Build history of the part. All positions in model axes, mm. Face numbers are marked on the shaded views. A direction names the side the tool comes from. Give positions to 0.01 mm unless a question says otherwise; leave off trailing zeros. Order: outer loops, then holes, each group sorted by start corner. A loop starts at its lowest first (then second) coordinate and runs counter-clockwise, first axis right, second up. Notation, with made-up numbers: (43, -29) -> (47, -29) arc R28 cw to (47, -5) -> close; hole circle Ø11 at (53, -22.75). An arc over 180 degrees is marked (long way). One line per question, with ' | ' between items. Start each with the question number.
(1) Cut at C-C (x = 62.5). Give the cut face in (y, z), then the cut area to 3 significant figures.
(2) Drill centre lines: L1, parallel to Y at x = -62, z = 8.5; L2, parallel to Z at x = -59, y = 38; L3, parallel to Z at x = 47.5, y = -47. Where is each one in solid material? Low to high. Write a range as from..to.
(3) Pin check, flat tips, straight feed: pin 1 Ø20 at (x, y) = (9, -26.5) entering from -Z; pin 2 Ø4.5 at (x, z) = (-2, 1.5) entering from -Y; pin 3 Ø16 at (x, y) = (93.5, 235) entering from +Z; pin 4 Ø6 at (y, z) = (109, -4) entering from +X. Stop position of each tip, or through.
(4) Cut at B-B (y = 129.5). Give the cut face in (x, z).
(5) Cut at A-A (z = -61). Give the cut face in (x, y).
(6) Cut at D-D (y = -14). Give the cut face in (x, z).
(7) Which spindle directions (+Z, -Z, +X, -X, +Y, -Y) get a long thin tool onto all of the face, cutting with end or side? Do the marked faces 1, 2, 3 and 4. Say none if no direction does.
from build123d import *

# Parameters (mm, degrees)
EXTRUDE_1_DEPTH = 4
SKETCH_11_W     = 156
SKETCH_11_H     = 90
EXTRUDE_2_DEPTH = 20
SKETCH_12_W     = 38
SKETCH_12_H     = 4
SKETCH_14_W     = 38
SKETCH_14_H     = 50
EXTRUDE_3_DEPTH = 20


with BuildPart() as part:
    # 草图1 → 凸台-拉伸1 (new body)
    with BuildSketch(Plane.XY):
        Polygon((-40, 0), (40, 0), (40, -160), (78, -160), (78, 0), (78, 50), (118, 90), (80, 90), (40, 50), (-40, 50), (-80, 90), (-118, 90), (-78, 50), (-78, 0), (-78, -160), (-40, -160), align=None)
    extrude(amount=EXTRUDE_1_DEPTH)

    # 草图11 → 凸台-拉伸2 (add)
    with BuildSketch(Plane.XY.offset(4)):
        with Locations((0, 5)):
            Rectangle(SKETCH_11_W, SKETCH_11_H)
    extrude(amount=EXTRUDE_2_DEPTH)

    # 扫描1: sweep along a path in 草图13
    with BuildLine(Plane(origin=(78, 0, 0), x_dir=(0, 0, -1), z_dir=(1, 0, 0))) as sweep_1_path:
        Line((-4, 90), (-4, 150))
        Line((-4, 150), (41, 227.942286341))
        Line((41, 227.942286341), (131, 227.942286341))
    # 草图12 → 扫描1 (sweep)
    with BuildSketch(Plane(origin=(0, 90, 0), x_dir=(1, 0, 0), z_dir=(0, 1, 0))):
        with Locations((-99, -2)):
            Rectangle(SKETCH_12_W, SKETCH_12_H)
        with Locations((99, -2)):
            Rectangle(SKETCH_12_W, SKETCH_12_H)
    sweep(path=sweep_1_path.line, transition=Transition.RIGHT)

    # 草图14 → 凸台-拉伸3 (add)
    with BuildSketch(Plane(origin=(0, 227.942286341, 0), x_dir=(1, 0, 0), z_dir=(0, 1, 0))):
        with Locations((-99, 106)):
            Rectangle(SKETCH_14_W, SKETCH_14_H)
        with Locations((99, 106)):
            Rectangle(SKETCH_14_W, SKETCH_14_H)
    extrude(amount=EXTRUDE_3_DEPTH)


solid = part.part
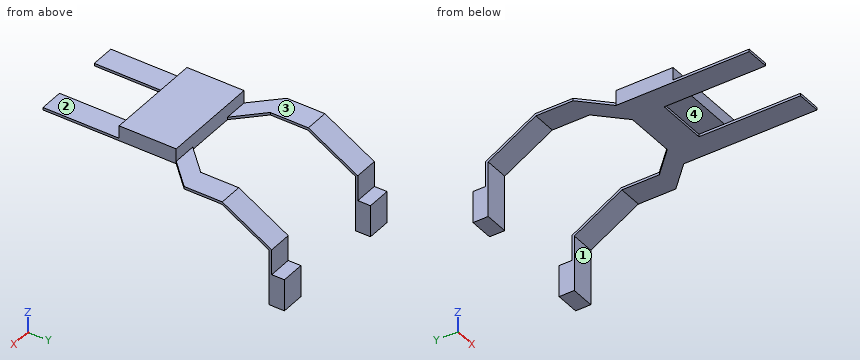
Result set:
1) outline: (-160, 0) -> (72.5, 0) -> (72.5, 4) -> (50, 4) -> (50, 24) -> (-40, 24) -> (-40, 4) -> (-160, 4) -> close | area: 2,730 mm2
2) L1: y = -40..50 | L2: z = 0..24 | L3: z = 0..4
3) pin 1: stops at z = 4 | pin 2: stops at y = 0 | pin 3: stops at z = -40.46 | pin 4: passes through
4) outline: (-118, 0) -> (-80, 0) -> (-80, 4) -> (-118, 4) -> close; (80, 0) -> (118, 0) -> (118, 4) -> (80, 4) -> close
5) outline: (-118, 223.94) -> (-80, 223.94) -> (-80, 227.94) -> (-118, 227.94) -> close; (80, 223.94) -> (118, 223.94) -> (118, 227.94) -> (80, 227.94) -> close
6) outline: (-78, 0) -> (-40, 0) -> (-40, 4) -> (40, 4) -> (40, 0) -> (78, 0) -> (78, 24) -> (-78, 24) -> close
7) face 1: -Z, +X, -X, -Y | face 2: +Z, +X, -X, -Y | face 3: +Z, +X, -X, +Y | face 4: -Z, -Y
